Build history of the part. All positions in model axes, mm. A direction names the side the tool comes from. Give positions to 0.01 mm unless a question says otherwise; leave off trailing zeros. Order: outer loops, then holes, each group sorted by start corner. A loop starts at its lowest first (then second) coordinate and runs counter-clockwise, first axis right, second up. Notation, with made-up numbers: (11.25, 57) - (31.25, 57) arc R24 ccw to (31.25, 76) - close; hole circle Ø9 at (78, -19.75). An arc over 180 degrees is marked (long way). Use a Markdown table: item, result.
from build123d import *

# Parameters (mm, degrees)
F0_W     = 152.4
F0_H     = 76.2
F1_DEPTH = 101.6
F3_DEPTH = 101.6
F5_DEPTH = 101.6
F6_W     = 63.5
F6_H     = 25.4
F7_DEPTH = 101.6
F9_DEPTH = 101.6


with BuildPart() as f1:
    # F0 (on Front) → F1 (new body)
    with BuildSketch(Plane.XZ):
        with Locations((-3.404423, -39.877999)):
            Rectangle(F0_W, F0_H)
    extrude(amount=-F1_DEPTH)

    # F2 (on face) → F3 (cut)
    with BuildSketch(Plane.XZ):
        Polygon((-25.510689, -1.777999), (-50.910689, -1.777999), (-50.910689, -14.477999), (-63.610689, -14.477999), (-63.610689, -27.177999), (-12.810689, -27.177999), (-12.810689, -14.477999), (-25.510689, -14.477999), align=None)
    extrude(amount=-F3_DEPTH, mode=Mode.SUBTRACT)

    # F4 (on face) → F5 (cut)
    with BuildSketch(Plane.YZ.offset(72.795577)):
        Polygon((73.393088, -49.326587), (22.593088, -49.326587), (34.413401, -77.977999), (59.813401, -77.977999), align=None)
    extrude(amount=-F5_DEPTH, mode=Mode.SUBTRACT)

    # F6 (on face) → F7 (cut)
    with BuildSketch(Plane.XZ):
        with Locations((41.045577, -14.477999)):
            Rectangle(F6_W, F6_H)
    extrude(amount=-F7_DEPTH, mode=Mode.SUBTRACT)

    # F8 (on face) → F9 (cut)
    with BuildSketch(Plane.XZ):
        Polygon((9.295577, -1.777999), (-8.107556, -1.777999), (9.295577, -27.177999), align=None)
    extrude(amount=-F9_DEPTH, mode=Mode.SUBTRACT)


solid = f1.part
1) Tool access for faces 1 (the flat face through (-17, 50, -1.778)), 2 (the flat face through (-25.511, 50, -8)), 3 (the flat face through (-57, 50, -14.478)), 4 (the flat face through (-79.604, 50, -40)), 5 (the flat face through (22.71, 66.51, -63.85)): list every direction of +Z, -Z, +X, -X, +Y, -Y with a clear straight run to the whole face (end or side of a thin tool).
Computed:
| item | result |
|---|---|
| face 1 | +Z, +X, -X, +Y, -Y |
| face 2 | +Z, +Y, -Y |
| face 3 | +Y, -Y |
| face 4 | +Z, -Z, -X, +Y, -Y |
| face 5 | +X |
2) Wall check: line 1 (Z direction, x = -24.5, y = 24); line 2 (Z direction, x = -15, y = 62); line 3 (Z direction, x = 56.5, y = 5.5). Give the ranges that are in metal, low to high. Write a range as from..to.
Computed:
| item | result |
|---|---|
| line 1 | z = -77.98..-52.74, -49.33..-27.18, -14.48..-1.78 |
| line 2 | z = -77.98..-73.36, -49.33..-27.18, -14.48..-1.78 |
| line 3 | z = -77.98..-27.18 |
3) Two-plate mould, pull along Y, no slides. Class faces 6 (the flat face through (-28.804, 48, -60)), 7 (the flat face through (-4, 101.6, -48)), 8 (the flat face through (-4, 0, -48)), 9 (the flat face through (-65, 50, -1.778)): +Y half, -Y half, draft (parallel to the pull), parting line (faces both ways), or undercut.
Computed:
| item | result |
|---|---|
| face 6 | undercut |
| face 7 | +Y half |
| face 8 | -Y half |
| face 9 | draft |
4) Pin check, flat tips, straight feed: P1, Ø12, axis at x = 34, y = 26, coming from the +Z side; P2, Ø15, axis at x = 14.5, y = 43, coming from the -Z side; P3, Ø10, axis at y = 31, z = -5, coming from the +X side. Stop position of each tip, or through.
Computed:
| item | result |
|---|---|
| P1 | stops at z = -27.18 |
| P2 | stops at z = -49.33 |
| P3 | stops at x = -2.47 |
5) Slice it at C-C (y = 80.5). Write the cut outline in (x, z), and give its area (3 significant figures).
Computed:
| item | result |
|---|---|
| outline | (-79.6, -77.98) - (72.8, -77.98) - (72.8, -27.18) - (9.3, -27.18) - (-8.11, -1.78) - (-25.51, -1.78) - (-25.51, -14.48) - (-12.81, -14.48) - (-12.81, -27.18) - (-63.61, -27.18) - (-63.61, -14.48) - (-50.91, -14.48) - (-50.91, -1.78) - (-79.6, -1.78) - close |
| area | 8,810 mm² |
6) Slice it at A-A (x = -52.5). Write the cut outline in (y, z), and give its area (3 significant figures).
Computed:
| item | result |
|---|---|
| outline | (0, -77.98) - (101.6, -77.98) - (101.6, -27.18) - (0, -27.18) - close; (0, -14.48) - (101.6, -14.48) - (101.6, -1.78) - (0, -1.78) - close |
| area | 6,450 mm² |
7) Slice it at B-B (z = -7). Write the cut outline in (x, y), and give its area (3 significant figures).
Computed:
| item | result |
|---|---|
| outline | (-79.6, 0) - (-50.91, 0) - (-50.91, 101.6) - (-79.6, 101.6) - close; (-25.51, 0) - (-4.53, 0) - (-4.53, 101.6) - (-25.51, 101.6) - close |
| area | 5,050 mm² |
8) Slice it at D-D (x = 61). Write the cut outline in (y, z), and give its area (3 significant figures).
Computed:
| item | result |
|---|---|
| outline | (0, -77.98) - (34.41, -77.98) - (22.59, -49.33) - (73.39, -49.33) - (59.81, -77.98) - (101.6, -77.98) - (101.6, -27.18) - (0, -27.18) - close |
| area | 4,070 mm² |
